Verification items for the finished model (mm, model axes). A direction names the side the tool comes from. Round coordinates to 2 decimals unless told otherwise and drop trailing zeros. Write each loop counter-clockwise with the first axis right and the second up, starting at its lowest first coordinate (ties: lowest second). Pieces come first, ordered by that corner, then holes. Notation, with made-up numbers: M -18.75,33 L 22.25,33 A14 cw 22.25,41 Z; hole C 37,41 d6. An arc over 180 degrees is marked long. One line per question, with ' | ' between items.
from build123d import *

# Parameters (mm, degrees)
ESQUISSE1_W        = 10
ESQUISSE1_H        = 5
ESQUISSE1_W_2      = 30
ESQUISSE1_W_3      = 5
BOSS_EXTRU_1_DEPTH = 5


with BuildPart() as part:
    # Esquisse1 → Boss.-Extru.1 (new body)
    with BuildSketch(Plane.XY):
        with BuildLine():
            Line((-55, 80), (-5, 80))
            ThreePointArc((-5, 80), (-1.464466094, 78.535533906), (0, 75))
            Line((0, 75), (0, 42.5))
            Line((0, 42.5), (-12.172703514, 42.5))
            ThreePointArc((-12.172703514, 42.5), (-15.374759815, 43.42586604), (-17.588591054, 45.917721519))
            ThreePointArc((-17.588591054, 45.917721519), (-43.75, 40), (-17.588591054, 34.082278481))
            ThreePointArc((-17.588591054, 34.082278481), (-15.374759815, 36.57413396), (-12.172703514, 37.5))
            Line((-12.172703514, 37.5), (0, 37.5))
            Line((0, 37.5), (0, 5))
            ThreePointArc((0, 5), (-1.464466094, 1.464466094), (-5, 0))
            Line((-5, 0), (-55, 0))
            ThreePointArc((-55, 0), (-58.535533906, 1.464466094), (-60, 5))
            Line((-60, 5), (-60, 75))
            ThreePointArc((-60, 75), (-58.535533906, 78.535533906), (-55, 80))
        make_face()
        with Locations((-50, 7.5)):
            Rectangle(ESQUISSE1_W, ESQUISSE1_H, mode=Mode.SUBTRACT)
        with Locations((-20, 7.5)):
            Rectangle(ESQUISSE1_W_2, ESQUISSE1_H, mode=Mode.SUBTRACT)
        with Locations((-20, 72.5)):
            Rectangle(ESQUISSE1_W_2, ESQUISSE1_H, mode=Mode.SUBTRACT)
        with Locations((-50, 72.5)):
            Rectangle(ESQUISSE1_W, ESQUISSE1_H, mode=Mode.SUBTRACT)
        with Locations((-30, 60.4)):
            Rectangle(ESQUISSE1_W_3, ESQUISSE1_H, mode=Mode.SUBTRACT)
        Polygon((-11.418018253, 53.615063509), (-8.918018253, 49.284936491), (-13.248145272, 46.784936491), (-15.748145272, 51.115063509), align=None, mode=Mode.SUBTRACT)
        Polygon((-8.918018253, 30.715063509), (-11.418018253, 26.384936491), (-15.748145272, 28.884936491), (-13.248145272, 33.215063509), align=None, mode=Mode.SUBTRACT)
        with Locations((-30, 19.6)):
            Rectangle(ESQUISSE1_W_3, ESQUISSE1_H, mode=Mode.SUBTRACT)
        Polygon((-48.581981747, 26.384936491), (-51.081981747, 30.715063509), (-46.751854728, 33.215063509), (-44.251854728, 28.884936491), align=None, mode=Mode.SUBTRACT)
        Polygon((-51.081981747, 49.284936491), (-48.581981747, 53.615063509), (-44.251854728, 51.115063509), (-46.751854728, 46.784936491), align=None, mode=Mode.SUBTRACT)
    extrude(amount=BOSS_EXTRU_1_DEPTH)


solid = part.part
1. Tool access check on faces 1 (the face through (-6, 42.5, 2)), 2 (the face through (-5, 72, 2)), 3 (the face through (-1, 2, 2)). Record the directions out of +Z, -Z, +X, -X, +Y, -Y that give a thin tool (end or side, any length) a straight path to the whole face; none if there is none.
Results:
face 1: +Z, -Z, +X | face 2: +Z, -Z | face 3: +Z, -Z, +X, -Y
2. Section check C-C, the plane y = 40. Record the cut outline in (x, z).
Results:
outline: M -60,0 L -43.75,0 L -43.75,5 L -60,5 Z
3. Thickness scan on line 1 (Y direction, x = -7, z = 1.6); line 2 (Y direction, x = -30, z = 3.4); line 3 (X direction, y = 6, z = 4.45). Record the ranges inside material, lowest first.
Results:
line 1: y = 0 to 5, 10 to 37.5, 42.5 to 70, 75 to 80 | line 2: y = 0 to 5, 10 to 17.1, 22.1 to 26.25, 53.75 to 57.9, 62.9 to 70, 75 to 80 | line 3: x = -60 to -55, -45 to -35, -5 to 0
4. Section check D-D, the plane x = -42. Record the cut outline in (y, z), then the cut area to 3 significant figures.
Results:
outline: M 0,0 L 33.29,0 L 33.29,5 L 0,5 Z; M 46.71,0 L 80,0 L 80,5 L 46.71,5 Z | area: 333 mm2
5. Section check B-B, the plane z = 2.9. Count the separate pieces of the cut face and the enclosed holes in it, then the cut area to 3 significant figures.
Results:
separate pieces: 1 | enclosed holes: 10 | area: 3,550 mm2
6. Section check A-A, the plane x = -30. Record the cut outline in (y, z), then the cut area to 4 significant figures.
Results:
outline: M 0,0 L 5,0 L 5,5 L 0,5 Z; M 10,0 L 17.1,0 L 17.1,5 L 10,5 Z; M 22.1,0 L 26.25,0 L 26.25,5 L 22.1,5 Z; M 53.75,0 L 57.9,0 L 57.9,5 L 53.75,5 Z; M 62.9,0 L 70,0 L 70,5 L 62.9,5 Z; M 75,0 L 80,0 L 80,5 L 75,5 Z | area: 162.5 mm2
7. Go/stop test with a flat-tipped pin: P1, Ø1.5, axis at x = -4, z = 3.5, coming from the +Y side. Record where the tip stops, or that it passes through.
Results:
P1: stops at y = 79.99
